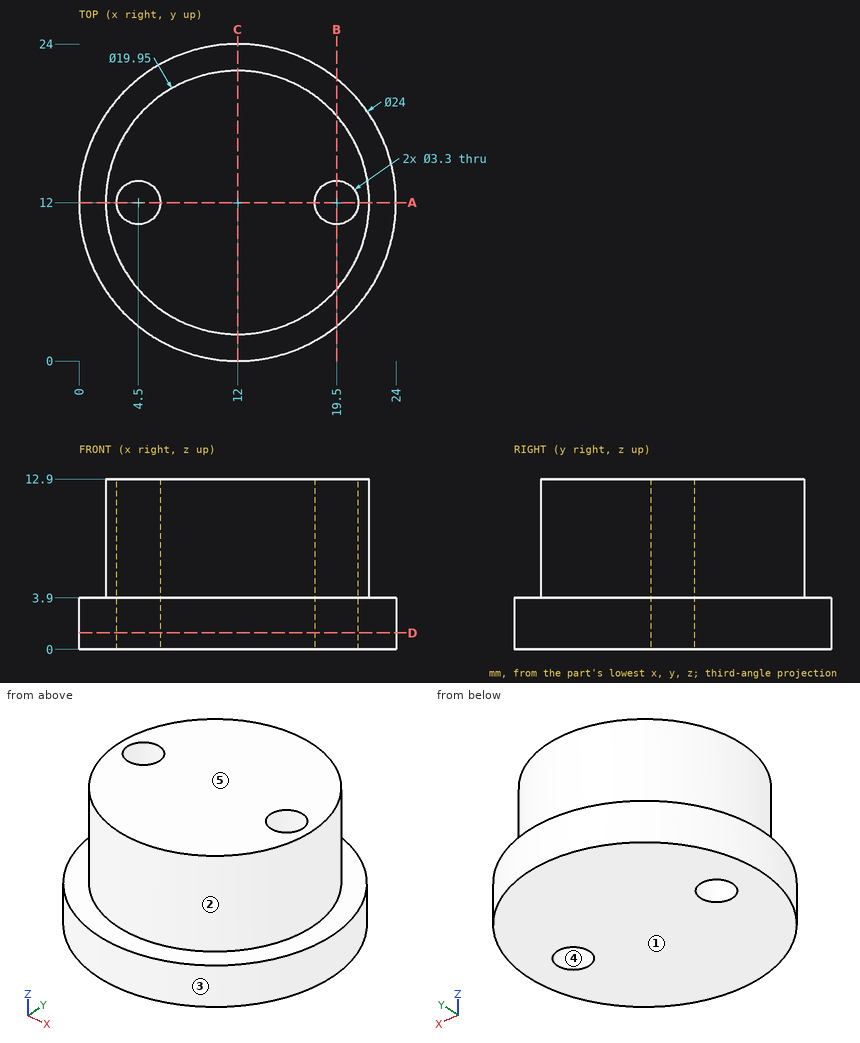
Could you check a few things on this drawing? It's one solid part, dimensions in mm from its lowest x, y, z. A direction names the side the tool comes from. Give positions to 0.01 mm unless a question says otherwise; leave off trailing zeros. Loops run counter-clockwise (first coordinate to the right, second up) from the corner with the lowest first, then second, coordinate; pieces in that order, holes last. Notation, with made-up numbers: M 21.5,-5 L 57.5,-5 A11 ccw 57.5,7 Z; hole C 27,82 d5. An arc over 180 degrees is marked long. Return JSON: item names as keys, results as strings.
Item 1: Imagine slicing it at B-B on x = 19.5. List the corners of the cut face in (y, z) for me.
A:
{"outline": "M 2.63,0 L 10.35,0 L 10.35,12.9 L 5.42,12.9 L 5.42,3.9 L 2.63,3.9 Z; M 13.65,0 L 21.37,0 L 21.37,3.9 L 18.58,3.9 L 18.58,12.9 L 13.65,12.9 Z"}
Item 2: I'm going to push flat-ended pins straight in: pin 1 Ø5 at (x, z) = (20, 2) entering from +Y; pin 2 Ø1.5 at (x, z) = (11, 9) entering from +Y; pin 3 Ø6 at (y, z) = (13.5, 9) entering from +X (3 decimals). Where does each tip first touch, or does it pass through?
A:
{"pin 1": "stops at y = 22.67", "pin 2": "stops at y = 21.97", "pin 3": "stops at x = 21.975"}
Item 3: Imagine slicing it at C-C on x = 12. List the corners of the cut face in (y, z) for me (3 decimals).
A:
{"outline": "M 0,0 L 24,0 L 24,3.9 L 21.975,3.9 L 21.975,12.9 L 2.025,12.9 L 2.025,3.9 L 0,3.9 Z"}
Item 4: On a 3-axis mill with a long thin cutter (end or side, diameter ignored), from which of +Z, -Z, +X, -X, +Y, -Y can I reach the whole of each face in a straight line? I mean the marked faces 1 and 2. Say none if no direction works.
A:
{"face 1": "-Z, +X, -X, +Y, -Y", "face 2": "+Z"}
Item 5: Imagine slicing it at A-A on y = 12. List the corners of the cut face in (x, z) for me (3 decimals).
A:
{"outline": "M 0,0 L 2.85,0 L 2.85,12.9 L 2.025,12.9 L 2.025,3.9 L 0,3.9 Z; M 6.15,0 L 17.85,0 L 17.85,12.9 L 6.15,12.9 Z; M 21.15,0 L 24,0 L 24,3.9 L 21.975,3.9 L 21.975,12.9 L 21.15,12.9 Z"}
Item 6: Imagine slicing it at D-D on z = 1.25. List the corners of the cut face in (x, y) for me.
A:
{"outline": "C 12,12 d24; hole C 4.5,12 d3.3; hole C 19.5,12 d3.3"}
Item 7: Please list where these lines run through material, in increasing order: line 1 (X direction, y = 11.5, z = 1.75); line 2 (Y direction, x = 4.25, z = 4); line 3 (Y direction, x = 19.5, z = 6.5).
A:
{"line 1": "x = 0.01 to 2.93, 6.07 to 17.93, 21.07 to 23.99", "line 2": "y = 5.72 to 10.37, 13.63 to 18.28", "line 3": "y = 5.42 to 10.35, 13.65 to 18.58"}
Item 8: Thinking about a two-plate mould opening in Y: for the marked faces 3, 4 and 5, which applies, released by +Y, released by -Y, zero draft, split by the parting line, or undercut?
A:
{"face 3": "split by the parting line", "face 4": "undercut", "face 5": "zero draft"}
